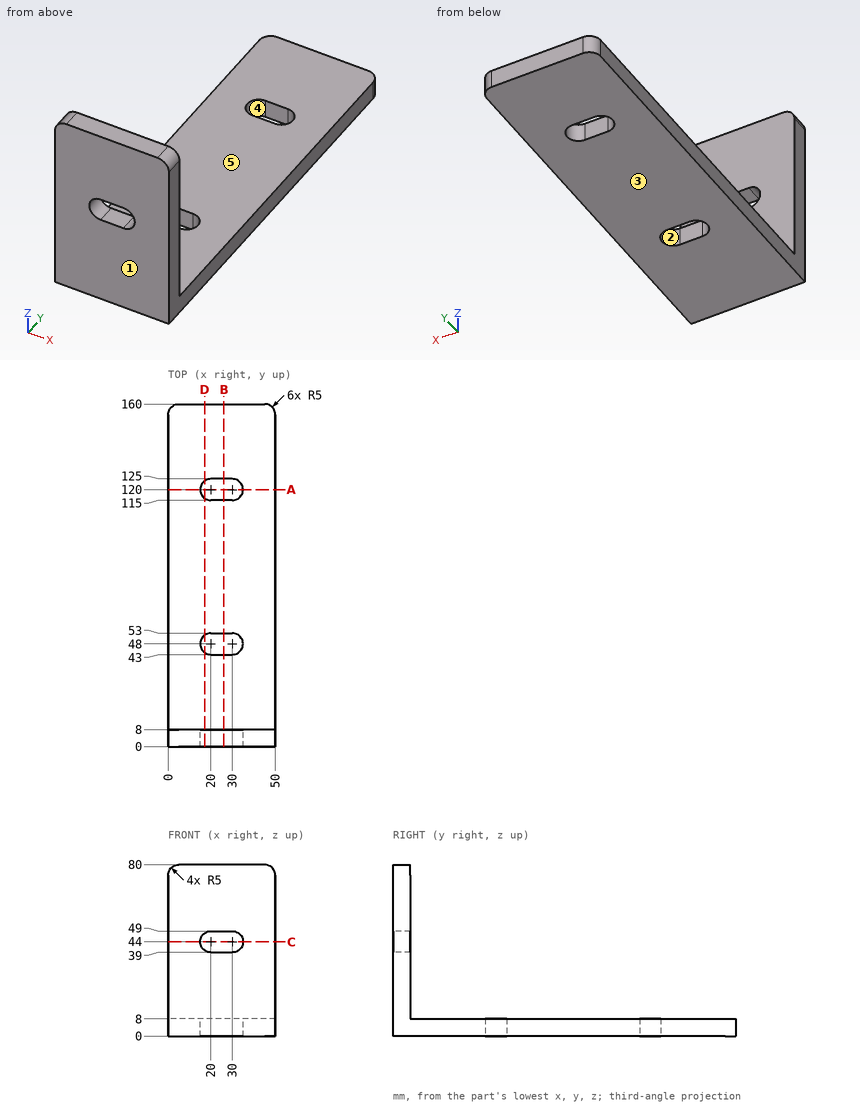
For this review, use the dimensioned drawing (mm, ordinates from the lowest corner) and the shaded views. A direction names the side the tool comes from. Coordinates: 2 decimals unless noted, no trailing zeros. Order: outer loops, then holes, each group sorted by start corner. A loop starts at its lowest first (then second) coordinate and runs counter-clockwise, first axis right, second up. Notation, with made-up numbers: M -16.75,-13.75 L 21.25,-13.75 A33 ccw 21.25,15.25 Z; hole C 60,13.25 d3. An arc over 180 degrees is marked long. Answer as a JSON object with one key per item and string values. Group by question number.
1) Add section D-D, the plane x = 17. Write out the cut boundary in (y, z), then the cut area to 3 significant figures.
2) Add section A-A, the plane y = 120. Write out the cut boundary in (x, z), then the cut area to 3 significant figures.
3) Add section B-B, the plane x = 26. Write out the cut boundary in (y, z), then the cut area to 3 significant figures.
4) Tool access review of the marked faces 3, 4 and 5: name each direction out of +Z, -Z, +X, -X, +Y, -Y from which nothing blocks a thin tool from reaching the whole face with its end or side.
5) For pin 1 (25 mm diameter, centred on x = 28.5, z = 61, fed in from +Y); pin 2 (25 mm diameter, centred on x = 16, y = 90, fed in from +Z), all flat-tipped, find the tip position at first contact; note any pin that passes through.
6) Mouldability with a two-part tool opening along X and no side actions: class the marked faces 1 and 2 as pulls with the +X half, pulls with the -X half, needs draft (parallel to the pull), parting line crosses it, or undercut.
7) Wall thickness on L1, parallel to Z at x = 18, y = 54: over which ranges is the line inside the solid? List them lowest first.
Computed values:
{
 "1": {"outline": "M 0,0 L 44,0 L 44,8 L 8,8 L 8,40 L 0,40 Z; M 0,48 L 8,48 L 8,80 L 0,80 Z; M 52,0 L 116,0 L 116,8 L 52,8 Z; M 124,0 L 160,0 L 160,8 L 124,8 Z", "area": "1,660 mm^2"},
 "2": {"outline": "M 0,0 L 15,0 L 15,8 L 0,8 Z; M 35,0 L 50,0 L 50,8 L 35,8 Z", "area": "240 mm^2"},
 "3": {"outline": "M 0,0 L 43,0 L 43,8 L 8,8 L 8,39 L 0,39 Z; M 0,49 L 8,49 L 8,80 L 0,80 Z; M 53,0 L 115,0 L 115,8 L 53,8 Z; M 125,0 L 160,0 L 160,8 L 125,8 Z", "area": "1,620 mm^2"},
 "4": {"face 3": "-Z, +X, -X, +Y, -Y", "face 4": "+Z, -Z", "face 5": "+Z, +X, -X, +Y"},
 "5": {"pin 1": "stops at y = 8", "pin 2": "stops at z = 8"},
 "6": {"face 1": "needs draft", "face 2": "undercut"},
 "7": {"L1": "z = 0 to 8"}
}
